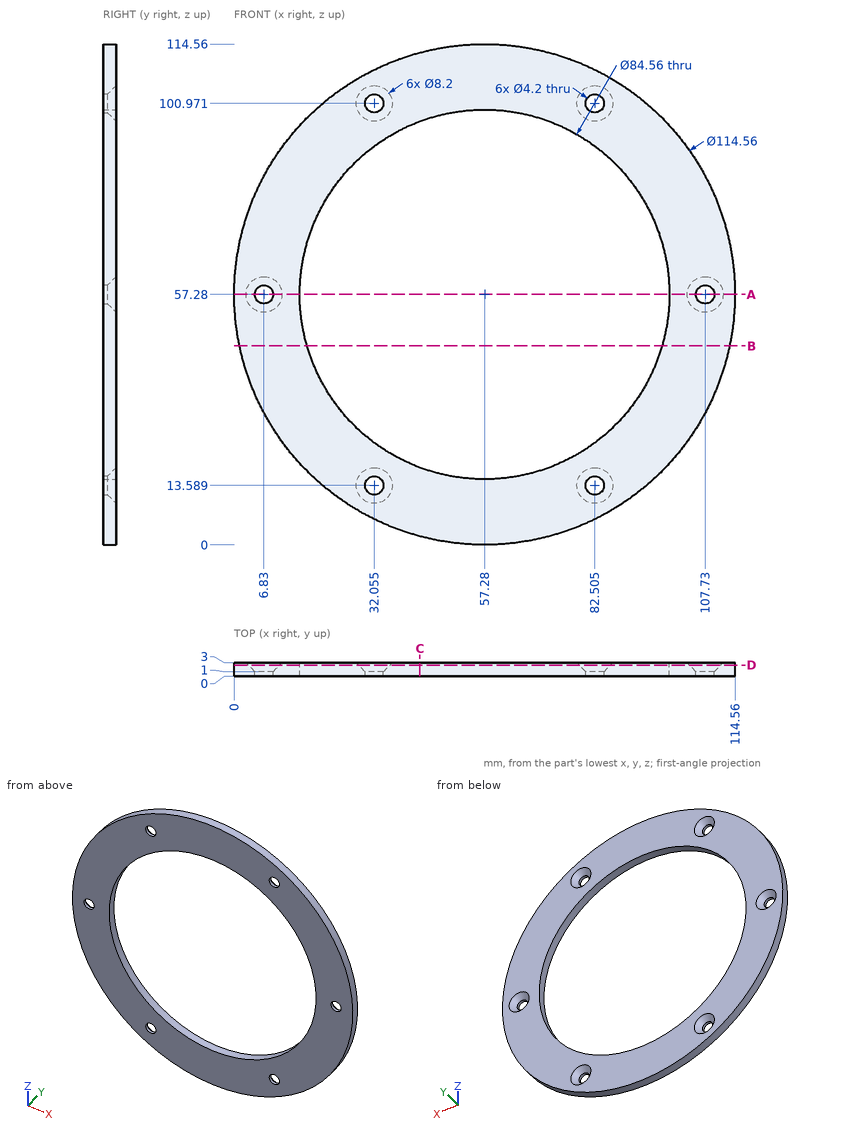
Here's the drawing with two shaded views (mm, measured from the low corner). I have some questions. Coordinates: 2 decimals unless noted, no trailing zeros. Write each loop counter-clockwise with the first axis right and the second up, starting at its lowest first coordinate (ties: lowest second). Pieces come first, ordered by that corner, then holes. Notation, with made-up numbers: M 32,45.25 L 73,45.25 A16 ccw 73,51.25 Z; hole C 9.5,16 d7. An arc over 180 degrees is marked long. Write item = value, one per line. Start each with the question number.
Q1. If we section it at D-D, the plane y = 2.5: Write out the boundary of the cut face in (x, z) (3 decimals).
Q2. I'm going to push flat-ended pins straight in: pin 1 (1.5 mm diameter, centred on y = 0.5, z = 55.5, fed in from -X); pin 2 (5.5 mm diameter, centred on x = 82.5, z = 13.59, fed in from +Y) (3 decimals); pin 3 (1 mm diameter, centred on y = 1.5, z = 22, fed in from +X). Where does each tip first touch, or does it pass through?
Q3. If we section it at C-C, the plane x = 42.5: Write out the boundary of the cut face in (y, z).
Q4. If we section it at B-B, the plane z = 45.5: Write out the boundary of the cut face in (x, y).
Q5. If I drill on L1, parallel to X at y = 0.2, z = 57.28; L2, parallel to X at y = 2, z = 57.5; L3, parallel to Z at x = 56, y = 1.3, over which ranges is the centre line in solid material (lowest first)? Write a range as [from, to].
Q6. If we section it at A-A, the plane z = 57.28: Write out the boundary of the cut face in (x, y).
Check sheet entries:
q1.outline = C 57.28,57.28 d114.56; hole C 6.83,57.28 d7.2; hole C 57.28,57.28 d84.56; hole C 32.055,13.589 d7.2; hole C 32.055,100.971 d7.2; hole C 82.505,13.589 d7.2; hole C 82.505,100.971 d7.2; hole C 107.73,57.28 d7.2
q2.pin_1 = 0.01
q2.pin_2 = 1.655
q2.pin_3 = 102.79
q3.outline = M 0,1.94 L 3,1.94 L 3,17.67 L 0,17.67 Z; M 0,96.89 L 3,96.89 L 3,112.62 L 0,112.62 Z
q4.outline = M 1.22,0 L 16.67,0 L 16.67,3 L 1.22,3 Z; M 97.89,0 L 113.34,0 L 113.34,3 L 97.89,3 Z
q5.L1 = [0, 4.73], [8.93, 15], [99.56, 105.63], [109.83, 114.56]
q5.L2 = [0, 3.74], [9.92, 15], [99.56, 104.64], [110.82, 114.56]
q5.L3 = [0.01, 15.02], [99.54, 114.55]
q6.outline = M 0,0 L 4.73,0 L 4.73,1 L 2.73,3 L 0,3 Z; M 8.93,0 L 15,0 L 15,3 L 10.93,3 L 8.93,1 Z; M 99.56,0 L 105.63,0 L 105.63,1 L 103.63,3 L 99.56,3 Z; M 109.83,0 L 114.56,0 L 114.56,3 L 111.83,3 L 109.83,1 Z
